Could you check a few things on this drawing? It's one solid part, dimensions in mm from its lowest x, y, z. Coordinates: 2 decimals unless noted, no trailing zeros. Write each loop counter-clockwise with the first axis right and the second up, starting at its lowest first coordinate (ties: lowest second). Pieces come first, ordered by that corner, then holes. Notation, with made-up numbers: M 1.25,81.5 L 22.25,81.5 A30 ccw 22.25,109.5 Z; hole C -18.75,19.25 d8. An arc over 180 degrees is marked long. Use a Markdown table: item, result.
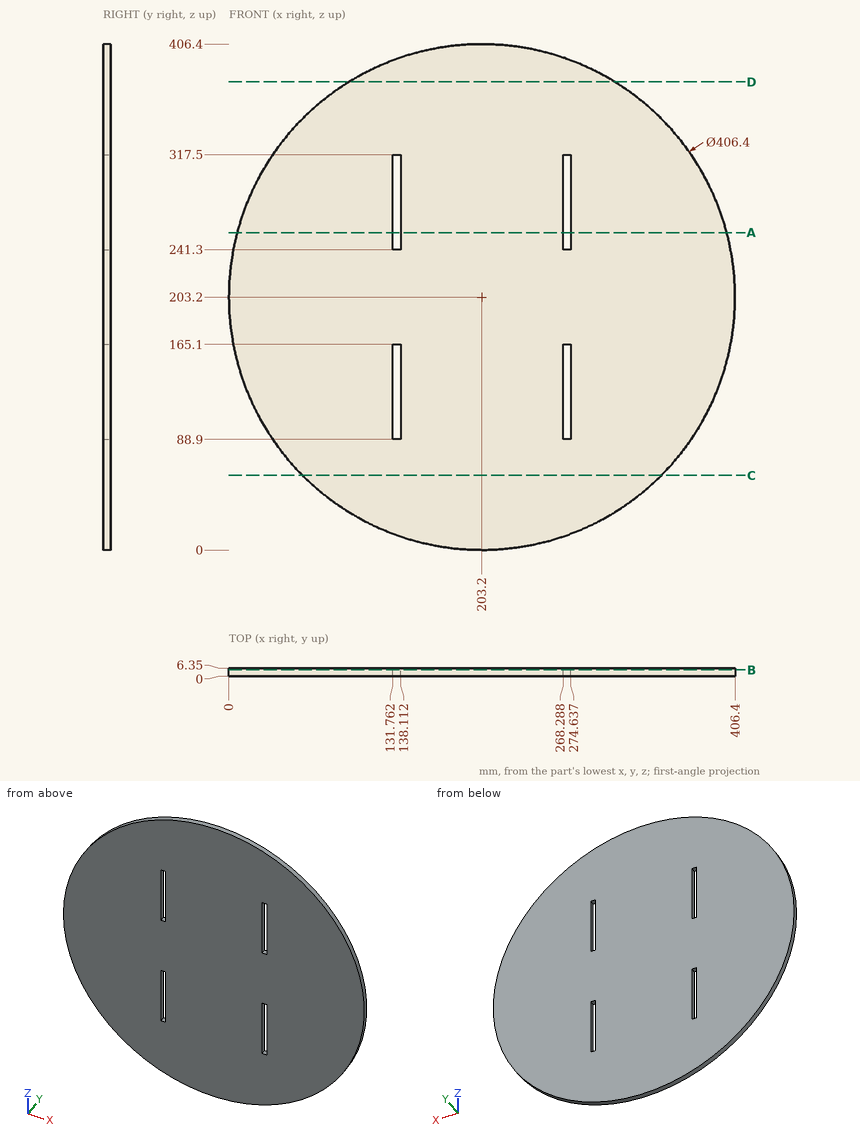
1. Suppose I cut it at C-C on z = 60. Write out the boundary of the cut face in (x, y), and give its area (3 significant figures).
Answers follow:
| item | result |
|---|---|
| outline | M 59.03,0 L 347.37,0 L 347.37,6.35 L 59.03,6.35 Z |
| area | 1,830 mm2 |
2. Will these pins go through, and if not, where does the flat tip stop? pin 1 Ø1.9 at (x, y) = (135, 4.5) entering from -Z; pin 2 Ø3 at (y, z) = (3.5, 286.5) entering from -X; pin 3 Ø3 at (y, z) = (4.5, 128.5) entering from -X.
Answers follow:
| item | result |
|---|---|
| pin 1 | stops at z = 11.45 |
| pin 2 | stops at x = 17.19 |
| pin 3 | stops at x = 13.64 |
3. I need wall thicknesses on probe 1 along X at (y, z) = (4.25, 147) (1 decimal); probe 2 along Z at (x, y) = (134, 4) (1 decimal); probe 3 along X at (y, z) = (3, 244.5). Which ranges of each line are inside material? Lowest first, please.
Answers follow:
| item | result |
|---|---|
| probe 1 | x = 7.9 to 131.8, 138.1 to 268.3, 274.6 to 398.5 |
| probe 2 | z = 12.1 to 88.9, 165.1 to 241.3, 317.5 to 394.3 |
| probe 3 | x = 4.24 to 131.76, 138.11 to 268.29, 274.64 to 402.16 |
4. Suppose I cut it at B-B on y = 5. Write out the boundary of the cut face in (x, z).
Answers follow:
| item | result |
|---|---|
| outline | C 203.2,203.2 d406.4; hole M 131.76,88.9 L 138.11,88.9 L 138.11,165.1 L 131.76,165.1 Z; hole M 131.76,241.3 L 138.11,241.3 L 138.11,317.5 L 131.76,317.5 Z; hole M 268.29,88.9 L 274.64,88.9 L 274.64,165.1 L 268.29,165.1 Z; hole M 268.29,241.3 L 274.64,241.3 L 274.64,317.5 L 268.29,317.5 Z |
5. Suppose I cut it at D-D on z = 376. Write out the boundary of the cut face in (x, y), and give its area (3 significant figures).
Answers follow:
| item | result |
|---|---|
| outline | M 96.29,0 L 310.11,0 L 310.11,6.35 L 96.29,6.35 Z |
| area | 1,360 mm2 |
6. Suppose I cut it at A-A on z = 255. Write out the boundary of the cut face in (x, y).
Answers follow:
| item | result |
|---|---|
| outline | M 6.71,0 L 131.76,0 L 131.76,6.35 L 6.71,6.35 Z; M 138.11,0 L 268.29,0 L 268.29,6.35 L 138.11,6.35 Z; M 274.64,0 L 399.69,0 L 399.69,6.35 L 274.64,6.35 Z |
